Build history of the part. All positions in model axes, mm. Face numbers are marked on the shaded views. A direction names the side the tool comes from. Round coordinates to 2 decimals unless told otherwise and drop trailing zeros. Write each loop counter-clockwise with the first axis right and the second up, starting at its lowest first coordinate (ties: lowest second). Pieces come first, ordered by that corner, then holes. Notation, with made-up numbers: (-4.75, 81) - (53.25, 81) arc R21 cw to (53.25, 106) - close; hole circle Ø7 at (21.25, 43.5). An arc over 180 degrees is marked (long way). Write each question's results on one line, items separated by ' | '.
from build123d import *

# Parameters (mm, degrees)
SKETCH1_R           = 4
BOSS_EXTRUDE1_DEPTH = 48
SKETCH2_R           = 4
SKETCH2_R_2         = 2.5
CUT_EXTRUDE1_DEPTH  = 14
CHAMFER1_SIZE       = 1


with BuildPart() as part:
    # Sketch1 → Boss-Extrude1 (new body)
    with BuildSketch(Plane(origin=(0, 0, 0), x_dir=(1, 0, 0), z_dir=(0, 1, 0))):
        with Locations(Location((0, 0, 0), (0, 0, 270))):
            Circle(SKETCH1_R)
    extrude(amount=BOSS_EXTRUDE1_DEPTH)

    # Sketch2 → Cut-Extrude1 (cut)
    with BuildSketch(Plane.XZ):
        with Locations(Location((0, 0, 0), (0, 0, 270))):
            Circle(SKETCH2_R)
        with Locations(Location((0, 0, 0), (0, 0, 270))):
            Circle(SKETCH2_R_2, mode=Mode.SUBTRACT)
    extrude(amount=-CUT_EXTRUDE1_DEPTH, mode=Mode.SUBTRACT)

    # Chamfer1
    chamfer1_edges = [part.edges().sort_by_distance(p)[0] for p in [
        (0, 48, -4),
    ]]
    chamfer(chamfer1_edges, length=CHAMFER1_SIZE)


solid = part.part
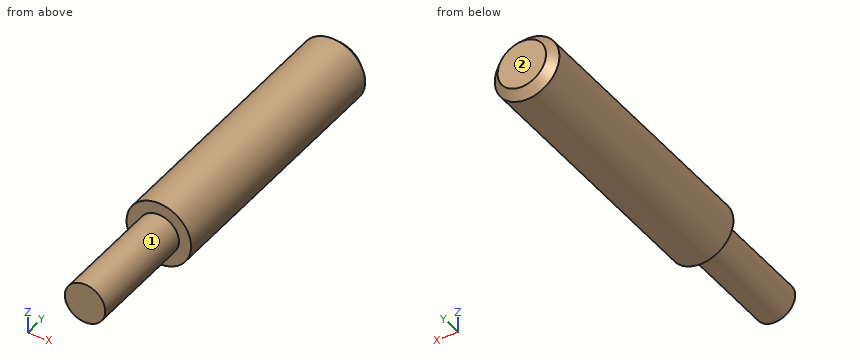
(1) Drill centre lines: probe 1 along Y at (x, z) = (0.25, -2.75); probe 2 along X at (y, z) = (23, 0.25); probe 3 along Z at (x, y) = (-1.5, 31.5). Where is each one in solid material? Low to high. Write a range as [from, to].
Worked answers:
probe 1: y = [14, 48] | probe 2: x = [-3.99, 3.99] | probe 3: z = [-3.71, 3.71]
(2) Tool access for the marked faces 1 and 2: list every direction of +Z, -Z, +X, -X, +Y, -Y with a clear straight run to the whole face (end or side of a thin tool).
Worked answers:
face 1: -Y | face 2: +Z, -Z, +X, -X, +Y
(3) Slice it at B-B, the plane x = 0. Write the cut outline in (y, z).
Worked answers:
outline: (0, -2.5) - (14, -2.5) - (14, -4) - (47, -4) - (48, -3) - (48, 3) - (47, 4) - (14, 4) - (14, 2.5) - (0, 2.5) - close
(4) Flat gauge pin, fed straight in: pin 1 Ø3 at (x, y) = (0.5, 21) entering from +Z. Where does the tip first touch, or does it go through?
Worked answers:
pin 1: stops at z = 4
(5) Slice it at A-A, the plane z = 0. Write the cut outline in (x, y), and give its area (3 significant figures).
Worked answers:
outline: (-4, 14) - (-2.5, 14) - (-2.5, 0) - (2.5, 0) - (2.5, 14) - (4, 14) - (4, 47) - (3, 48) - (-3, 48) - (-4, 47) - close | area: 341 mm2
(6) Slice it at D-D, the plane y = 5. Write the cut outline in (x, z), and give its area (3 significant figures).
Worked answers:
outline: circle Ø5 at (0, 0) | area: 19.6 mm2
(7) Slice it at C-C, the plane y = 44.5. Write the cut outline in (x, z).
Worked answers:
outline: circle Ø8 at (0, 0)
